Here's how the part is built. I have some questions about the finished solid (model axes, mm). Coordinates: 2 decimals unless noted, no trailing zeros. Write each loop counter-clockwise with the first axis right and the second up, starting at its lowest first coordinate (ties: lowest second). Pieces come first, ordered by that corner, then holes. Notation, with made-up numbers: (0, 39.25) -> (8, 39.25) arc R18 cw to (8, 59.25) -> close; hole circle Ø9 at (-15.5, 55.5). An arc over 180 degrees is marked (long way). Put each result on its own line as item: value. Start each with the question number.
Item 1: I want a section at A-A, the plane x = -46.5. List the corners of the cut face in (y, z) for me, then the cut area to 3 significant figures.
Item 2: I want a section at D-D, the plane z = 1.7. State how many separate pieces and enclosed holes the cut face has, then the cut area to 3 significant figures.
Item 3: I need wall thicknesses on line 1 (X direction, y = -8.5, z = 3.15); line 2 (X direction, y = -24, z = 2); line 3 (X direction, y = -13.5, z = 1.9). Which ranges of each line are inside material? Lowest first, please. Write a range as [from, to].
Item 4: I want a section at B-B, the plane y = -16. List the corners of the cut face in (x, z) for me.
Item 5: I want a section at C-C, the plane x = 30.5. List the corners of the cut face in (y, z) for me, then the cut area to 3 significant figures.
Item 6: For pin 1 (1 mm diameter, centred on y = -23.5, z = 4.5, fed in from -X); pin 2 (2 mm diameter, centred on x = -8.5, z = 4.5, fed in from +Y); pin 3 (1 mm diameter, centred on x = -24.5, z = 4, fed in from -Y), each with a flat end and sliding along its axis, tell me the tip position at first contact or that it passes through.
from build123d import *

# Parameters (mm, degrees)
SKETCH_1_W          = 144
SKETCH_1_H          = 68
EXTRUDE_1_DEPTH     = 5
SKETCH_2_R          = 1.25
CUT_EXTRUDE_1_DEPTH = 87.344031922
SKETCH_3_W          = 72
SKETCH_3_H          = 26
CUT_EXTRUDE_2_DEPTH = 87.344031922
SKETCH_5_R          = 1.25
CUT_EXTRUDE_3_DEPTH = 87.344031922
CUT_EXTRUDE_4_DEPTH = 87.344031922
SKETCH_7_R          = 4
CUT_EXTRUDE_5_DEPTH = 87.344031922
SKETCH_8_R          = 2.5
CUT_EXTRUDE_6_DEPTH = 87.344031922
FILLET_1_R          = 2


with BuildPart() as part:
    # Эскиз1 → Бобышка-Вытянуть1 (new body)
    with BuildSketch(Plane.XY):
        with Locations((3.041351056, -8.41565136)):
            Rectangle(SKETCH_1_W, SKETCH_1_H)
    extrude(amount=EXTRUDE_1_DEPTH)

    # Эскиз2 → Вырез-Вытянуть1 (cut, through all)
    with BuildSketch(Plane.XY.offset(5)):
        with Locations((-58.958648944, 7.08434864)):
            Circle(SKETCH_2_R)
        with Locations((-58.958648944, -23.91565136)):
            Circle(SKETCH_2_R)
        with Locations((16.041351056, 7.08434864)):
            Circle(SKETCH_2_R)
        with Locations((16.041351056, -23.91565136)):
            Circle(SKETCH_2_R)
    extrude(amount=-CUT_EXTRUDE_1_DEPTH, mode=Mode.SUBTRACT)

    # Эскиз3 → Вырез-Вытянуть2 (cut, through all)
    with BuildSketch(Plane.XY.offset(5)):
        with Locations((-21.458648944, -8.41565136)):
            Rectangle(SKETCH_3_W, SKETCH_3_H)
    extrude(amount=-CUT_EXTRUDE_2_DEPTH, mode=Mode.SUBTRACT)

    # Эскиз5 → Вырез-Вытянуть3 (cut, through all)
    with BuildSketch(Plane.XY.offset(5)):
        with Locations((22.041351056, -24.16565136)):
            Circle(SKETCH_5_R)
        with Locations((65.041351056, -24.16565136)):
            Circle(SKETCH_5_R)
        with Locations((65.041351056, 7.33434864)):
            Circle(SKETCH_5_R)
        with Locations((22.041351056, 7.33434864)):
            Circle(SKETCH_5_R)
    extrude(amount=-CUT_EXTRUDE_3_DEPTH, mode=Mode.SUBTRACT)

    # Эскиз6 → Вырез-Вытянуть4 (cut, through all)
    with BuildSketch(Plane.XY.offset(5)):
        with BuildLine():
            Line((27.541351056, -8.016688712), (34.541351056, -8.016688712))
            ThreePointArc((34.541351056, -8.016688712), (35.190313704, -8.66565136), (34.541351056, -9.314614008))
            Line((34.541351056, -9.314614008), (27.541351056, -9.314614008))
            ThreePointArc((27.541351056, -9.314614008), (26.892388408, -8.66565136), (27.541351056, -8.016688712))
        make_face()
        with BuildLine():
            Line((27.541351056, -5.016688712), (34.541351056, -5.016688712))
            ThreePointArc((34.541351056, -5.016688712), (35.190313704, -5.66565136), (34.541351056, -6.314614008))
            Line((34.541351056, -6.314614008), (27.541351056, -6.314614008))
            ThreePointArc((27.541351056, -6.314614008), (26.892388408, -5.66565136), (27.541351056, -5.016688712))
        make_face()
        with BuildLine():
            Line((27.541351056, -2.016688712), (34.541351056, -2.016688712))
            ThreePointArc((34.541351056, -2.016688712), (35.190313704, -2.66565136), (34.541351056, -3.314614008))
            Line((34.541351056, -3.314614008), (27.541351056, -3.314614008))
            ThreePointArc((27.541351056, -3.314614008), (26.892388408, -2.66565136), (27.541351056, -2.016688712))
        make_face()
    extrude(amount=-CUT_EXTRUDE_4_DEPTH, mode=Mode.SUBTRACT)

    # Эскиз7 → Вырез-Вытянуть5 (cut, through all)
    with BuildSketch(Plane.XY.offset(5)):
        with Locations((52.341351056, -8.41565136)):
            Circle(SKETCH_7_R)
    extrude(amount=-CUT_EXTRUDE_5_DEPTH, mode=Mode.SUBTRACT)

    # Эскиз8 → Вырез-Вытянуть6 (cut, through all)
    with BuildSketch(Plane.XY.offset(5)):
        with Locations((-60.958648944, 17.58434864)):
            Circle(SKETCH_8_R)
        with Locations((67.041351056, 17.58434864)):
            Circle(SKETCH_8_R)
        with Locations((67.041351056, -34.41565136)):
            Circle(SKETCH_8_R)
        with Locations((-60.958648944, -34.41565136)):
            Circle(SKETCH_8_R)
    extrude(amount=-CUT_EXTRUDE_6_DEPTH, mode=Mode.SUBTRACT)

    # Скругление1
    fillet_1_edges = [part.edges().sort_by_distance(p)[0] for p in [
        (75.041351056, -8.41565136, 5),
        (3.041351056, 25.58434864, 5),
        (-68.958648944, -8.41565136, 5),
        (3.041351056, -42.41565136, 5),
    ]]
    fillet(fillet_1_edges, radius=FILLET_1_R)


solid = part.part
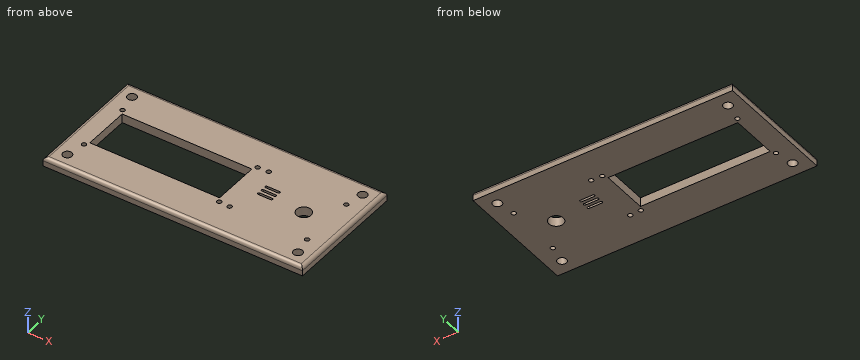
Calculated:
1. outline: (-42.42, 0) -> (-21.42, 0) -> (-21.42, 5) -> (-40.42, 5) arc R2 ccw to (-42.42, 3) -> close; (4.58, 0) -> (25.58, 0) -> (25.58, 3) arc R2 ccw to (23.58, 5) -> (4.58, 5) -> close
1. area: 208 mm2
2. separate pieces: 1
2. enclosed holes: 17
2. area: 7,720 mm2
3. line 1: x = [-68.95, -57.46], [14.54, 26.91], [35.17, 48.34], [56.34, 75.04]
3. line 2: x = [-68.96, -60.21], [-57.71, 14.79], [17.29, 20.8], [23.28, 63.8], [66.28, 75.04]
3. line 3: x = [-68.96, -57.46], [14.54, 75.04]
4. outline: (-68.96, 0) -> (-57.46, 0) -> (-57.46, 5) -> (-66.96, 5) arc R2 ccw to (-68.96, 3) -> close; (14.54, 0) -> (75.04, 0) -> (75.04, 3) arc R2 ccw to (73.04, 5) -> (14.54, 5) -> close
5. outline: (-42.42, 0) -> (-9.31, 0) -> (-9.31, 5) -> (-40.42, 5) arc R2 ccw to (-42.42, 3) -> close; (-8.02, 0) -> (-6.31, 0) -> (-6.31, 5) -> (-8.02, 5) -> close; (-5.02, 0) -> (-3.31, 0) -> (-3.31, 5) -> (-5.02, 5) -> close; (-2.02, 0) -> (25.58, 0) -> (25.58, 3) arc R2 ccw to (23.58, 5) -> (-2.02, 5) -> close
5. area: 319 mm2
6. pin 1: stops at x = -68.69
6. pin 2: stops at y = 25.52
6. pin 3: stops at y = -42.35
